Check sheet for the drawn part. Datum: minimum x, y, z corner. Units: mm. Coordinates: 2 decimals unless noted, no trailing zeros. Write each loop counter-clockwise with the first axis right and the second up, starting at its lowest first coordinate (ties: lowest second). Pieces come first, ordered by that corner, then holes. Notation, with made-up numbers: (87.25, -11.75) -> (95.25, -11.75) arc R25 cw to (95.25, 14.25) -> close; hole circle Ø10 at (-3, 33.25). An arc over 180 degrees is marked (long way). Write each question's results on one line, items separated by ' | '. Start each with the question number.
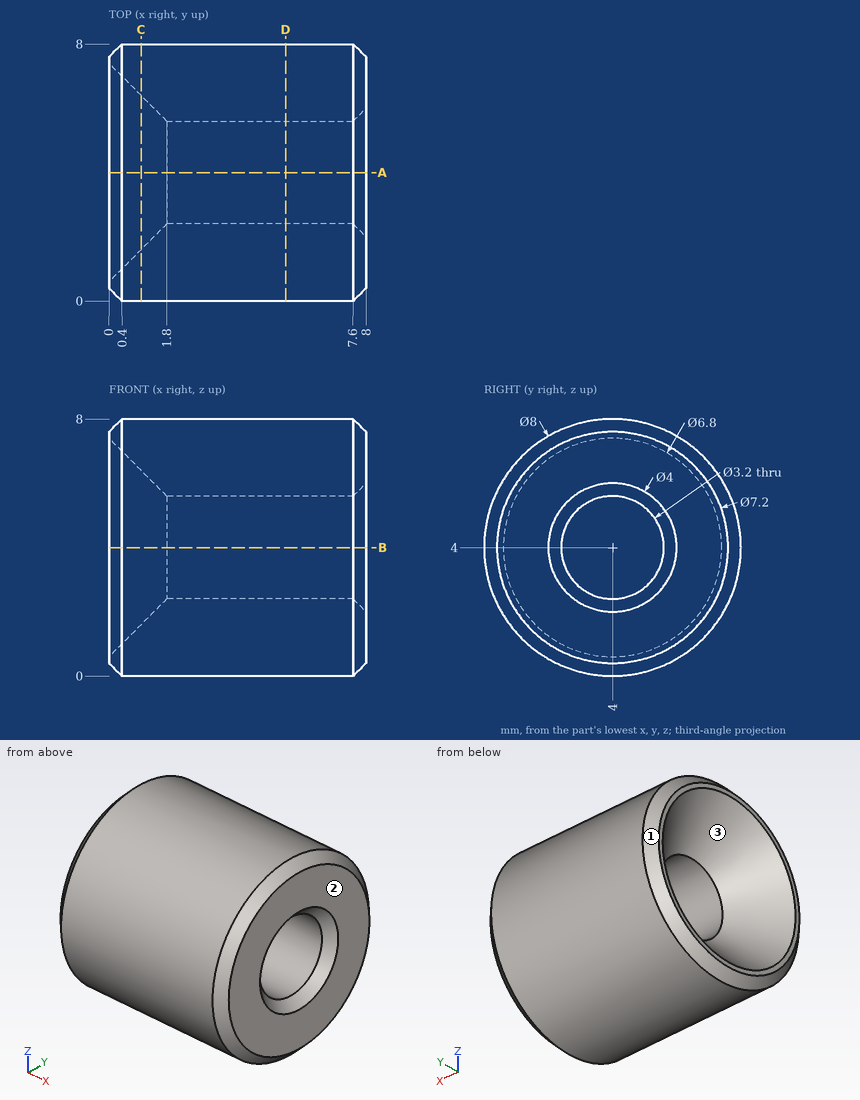
1. Sectioned sample at C-C on x = 1. Record the cut outline in (y, z).
2. Mould release check, pull along Z, two halves, no side actions. Record for the marked faces 1, 2 and 3: +Z half, -Z half, draft (parallel to the pull), parting line (faces both ways), or undercut.
3. Depth check by flat-ended pin: pin 1 Ø2 at (x, y) = (4, 1) entering from +Z. Enter the tip coordinate at first touch or a pass-through.
4. Material ranges on probe 1 along Z at (x, y) = (3.35, 4); probe 2 along Y at (x, z) = (2.25, 5); probe 3 along Y at (x, z) = (1, 2), recorded low to high. Write a range as from..to.
5. Sectioned sample at D-D on x = 5.5. Record the cut outline in (y, z), plus the area to 3 significant figures.
6. Sectioned sample at A-A on y = 4. Record the cut outline in (x, z).
Computed values:
1) outline: circle Ø8 at (4, 4); hole circle Ø4.8 at (4, 4)
2) face 1: parting line | face 2: draft | face 3: undercut
3) pin 1: stops at z = 7.46
4) probe 1: z = 0..2.4, 5.6..8 | probe 2: y = 0.13..2.75, 5.25..7.87 | probe 3: y = 0.54..2.67, 5.33..7.46
5) outline: circle Ø8 at (4, 4); hole circle Ø3.2 at (4, 4) | area: 42.2 mm^2
6) outline: (0, 0.4) -> (0.4, 0) -> (7.6, 0) -> (8, 0.4) -> (8, 2) -> (7.6, 2.4) -> (1.8, 2.4) -> (0, 0.6) -> close; (0, 7.4) -> (1.8, 5.6) -> (7.6, 5.6) -> (8, 6) -> (8, 7.6) -> (7.6, 8) -> (0.4, 8) -> (0, 7.6) -> close
